The listing builds one solid part. Answer for the finished solid, in the listing's coordinates (mm). A direction names the side the tool comes from. Give positions to 0.01 mm unless a question says otherwise; leave off trailing zeros. Order: outer loops, then holes, each group sorted by start corner. A loop starts at its lowest first (then second) coordinate and runs counter-clockwise, first axis right, second up. Notation, with made-up numbers: (56.5, -4.75) - (63.5, -4.75) arc R32 cw to (63.5, 21.25) - close; hole circle Ø11 at (78.5, 1.5). An arc over 180 degrees is marked (long way). Use CSV: the item, a comma, the result in double quotes.
```python
from build123d import *

# Parameters (mm, degrees)
F1_DEPTH = 40
F2_R     = 1.5
F3_DEPTH = 25
F4_R     = 2.5
F5_DEPTH = 25
F6_R     = 2.5
F7_DEPTH = 25


with BuildPart() as f1:
    # F0 (on Front) → F1 (new body)
    with BuildSketch(Plane.XZ):
        Polygon((-13.5, 0), (0, 0), (13.5, 0), (13.5, -18), (31.5, -18), (31.5, -15), (16.5, -15), (16.5, 3), (0, 3), (-16.5, 3), (-16.5, -15), (-31.5, -15), (-31.5, -18), (-13.5, -18), align=None)
    extrude(amount=F1_DEPTH)

    # F2 (on face) → F3 (cut)
    with BuildSketch(Plane.XY.offset(3)):
        with Locations((-10, -10)):
            Circle(F2_R)
        with Locations((10, -10)):
            Circle(F2_R)
        with Locations((10, -30)):
            Circle(F2_R)
        with Locations((-10, -30)):
            Circle(F2_R)
    extrude(amount=-F3_DEPTH, mode=Mode.SUBTRACT)

    # F4 (on face) → F5 (cut)
    with BuildSketch(Plane.XY.offset(-15)):
        with Locations((-24, -30)):
            Circle(F4_R)
        with Locations((-24, -20)):
            Circle(F4_R)
        with Locations((-24, -10)):
            Circle(F4_R)
    extrude(amount=-F5_DEPTH, mode=Mode.SUBTRACT)

    # F6 (on face) → F7 (cut)
    with BuildSketch(Plane.XY.offset(-15)):
        with Locations((24, -30)):
            Circle(F6_R)
        with Locations((24, -20)):
            Circle(F6_R)
        with Locations((24, -10)):
            Circle(F6_R)
    extrude(amount=-F7_DEPTH, mode=Mode.SUBTRACT)


solid = f1.part
```
Item 1: The part is cut by section C-C (y = -20). Give the vertices of the cut face in (x, z).
Taken from the geometry:
outline,"(-31.5, -18) - (-26.5, -18) - (-26.5, -15) - (-31.5, -15) - close; (-21.5, -18) - (-13.5, -18) - (-13.5, 0) - (13.5, 0) - (13.5, -18) - (21.5, -18) - (21.5, -15) - (16.5, -15) - (16.5, 3) - (-16.5, 3) - (-16.5, -15) - (-21.5, -15) - close; (26.5, -18) - (31.5, -18) - (31.5, -15) - (26.5, -15) - close"
Item 2: The part is cut by section A-A (z = -13). Give the vertices of the cut face in (x, y).
Taken from the geometry:
outline,"(-16.5, -40) - (-13.5, -40) - (-13.5, 0) - (-16.5, 0) - close; (13.5, -40) - (16.5, -40) - (16.5, 0) - (13.5, 0) - close"
Item 3: The part is cut by section B-B (x = 24). Give the vertices of the cut face in (y, z).
Taken from the geometry:
outline,"(-40, -18) - (-32.5, -18) - (-32.5, -15) - (-40, -15) - close; (-27.5, -18) - (-22.5, -18) - (-22.5, -15) - (-27.5, -15) - close; (-17.5, -18) - (-12.5, -18) - (-12.5, -15) - (-17.5, -15) - close; (-7.5, -18) - (0, -18) - (0, -15) - (-7.5, -15) - close"
Item 4: The part is cut by section D-D (z = 1.75). Give the vertices of the cut face in (x, y).
Taken from the geometry:
outline,"(-16.5, -40) - (16.5, -40) - (16.5, 0) - (-16.5, 0) - close; hole circle Ø3 at (-10, -30); hole circle Ø3 at (-10, -10); hole circle Ø3 at (10, -30); hole circle Ø3 at (10, -10)"
Item 5: Find the intervals of material crossed by line 1 along Y through (x, z) = (24, -15.85); line 2 along Y through (x, z) = (10, 1.9); line 3 along X through (y, z) = (-5, -9.75), in increasing order.
Taken from the geometry:
line 1,"-40 to -32.5, -27.5 to -22.5, -17.5 to -12.5, -7.5 to 0"
line 2,"-40 to -31.5, -28.5 to -11.5, -8.5 to 0"
line 3,"-16.5 to -13.5, 13.5 to 16.5"
Item 6: Each of these flat-tipped pins is pushed along its axis until it touches: pin 1 (5.5 mm diameter, centred on y = -21, z = -10.5, fed in from -X); pin 2 (1.5 mm diameter, centred on y = -21.5, z = -0.5, fed in from +X); pin 3 (12 mm diameter, centred on x = 25.5, y = -12.5, fed in from +Z). Where does it stop, or does it pass through?
Taken from the geometry:
pin 1,"x = -16.5"
pin 2,"x = 16.5"
pin 3,"z = -15"
Item 7: Which of the six approach directions +Z, -Z, +X, -X, +Y, -Y give full straight-line access (tool end or side, diameter ignored) to faces 4 (the face through (-27, -20, -15)), 5 (the face through (-13.5, -20, -9)), 6 (the face through (16.5, -20, -6))?
Taken from the geometry:
face 4,"+Z, -X, +Y, -Y"
face 5,"-Z, +Y, -Y"
face 6,"+Z, +X, +Y, -Y"
Item 8: The mould has two halves that part along Y. Classify faces 1 (the face through (-0.1, 0, 0.3)), 2 (the face through (20, -20, -18)), 3 (the face through (-26, -11.5, -16.5)): +Y half, -Y half, draft (parallel to the pull), parting line (faces both ways), or undercut.
Taken from the geometry:
face 1,"+Y half"
face 2,"draft"
face 3,"undercut"
